Can you work these out from the model? Positions are in its coordinate system, mm. Coordinates: 2 decimals unless noted, no trailing zeros. Loops run counter-clockwise (first coordinate to the right, second up) from the corner with the lowest first, then second, coordinate; pieces in that order, holes last. Notation, with made-up numbers: (-24, -35.75) -> (15, -35.75) arc R33 cw to (15, -0.75) -> close; hole circle Ø11 at (-36.5, 14). An arc over 180 degrees is marked (long way). Use one line per item in the form item = value. Start each with the question number.
(1) Imagine slicing it at A-A (y = -23). List the corners of the cut face in (x, z) for me.
(2) Imagine slicing it at B-B (x = 47.5). List the corners of the cut face in (y, z) for me.
(3) I'm going to push a flat-ended pin straight in: pin 1 (8 mm diameter, centred on x = -12, y = -1.5, fed in from +Z). Where does the tip first touch, or does it pass through?
(4) Imagine slicing it at C-C (z = 1.5). State how many separate pieces and enclosed holes the cut face has, plus the area to 4 significant figures.
(5) Thinking about a two-plate mould opening in Y: for faces 1 (the flat face through (30, 7.5, 3)), 2 (the flat face through (-1, 0, 5)), which applies, released by +Y, released by -Y, zero draft, split by the parting line, or undercut?
(6) I need wall thicknesses on line 1 (Y direction, x = 26, z = 1.75). Which ranges of the line are inside material? Lowest first, please. Write a range as [from, to].
```python
from build123d import *

# Parameters (mm, degrees)
SKETCH_1_W                  = 125
SKETCH_1_H                  = 65
EXTRUDE_1_DEPTH             = 5
SKETCH_2_W                  = 15
SKETCH_2_H                  = 15
CUT_EXTRUDE_1_DEPTH         = 5
PATTERN_LINEAR_1_COUNT      = 6
PATTERN_LINEAR_1_PITCH      = 20
PATTERN_LINEAR_1_COUNT_DIR2 = 3
PATTERN_LINEAR_1_PITCH_DIR2 = 20


with BuildPart() as part:
    # 草图1 → 凸台-拉伸1 (new body)
    with BuildSketch(Plane.XY):
        Rectangle(SKETCH_1_W, SKETCH_1_H)
    extrude(amount=EXTRUDE_1_DEPTH)

    # 草图2 → 切除-拉伸1 (cut)
    with BuildSketch(Plane.XY.offset(5)):
        with Locations((-50, 20)):
            Rectangle(SKETCH_2_W, SKETCH_2_H)
    cut_extrude_1 = extrude(amount=-CUT_EXTRUDE_1_DEPTH, mode=Mode.SUBTRACT)

    # 阵列(线性)1: Cut-Extrude 1 6 × 3
    with Locations(*[(i * PATTERN_LINEAR_1_PITCH, -j * PATTERN_LINEAR_1_PITCH_DIR2, 0) for i in range(PATTERN_LINEAR_1_COUNT) for j in range(PATTERN_LINEAR_1_COUNT_DIR2) if (i, j) != (0, 0)]):
        add(cut_extrude_1, mode=Mode.SUBTRACT)


solid = part.part
```
Worked out:
q1.outline = (-62.5, 0) -> (-57.5, 0) -> (-57.5, 5) -> (-62.5, 5) -> close; (-42.5, 0) -> (-37.5, 0) -> (-37.5, 5) -> (-42.5, 5) -> close; (-22.5, 0) -> (-17.5, 0) -> (-17.5, 5) -> (-22.5, 5) -> close; (-2.5, 0) -> (2.5, 0) -> (2.5, 5) -> (-2.5, 5) -> close; (17.5, 0) -> (22.5, 0) -> (22.5, 5) -> (17.5, 5) -> close; (37.5, 0) -> (42.5, 0) -> (42.5, 5) -> (37.5, 5) -> close; (57.5, 0) -> (62.5, 0) -> (62.5, 5) -> (57.5, 5) -> close
q2.outline = (-32.5, 0) -> (-27.5, 0) -> (-27.5, 5) -> (-32.5, 5) -> close; (-12.5, 0) -> (-7.5, 0) -> (-7.5, 5) -> (-12.5, 5) -> close; (7.5, 0) -> (12.5, 0) -> (12.5, 5) -> (7.5, 5) -> close; (27.5, 0) -> (32.5, 0) -> (32.5, 5) -> (27.5, 5) -> close
q3.pin_1 = through
q4.separate_pieces = 1
q4.enclosed_holes = 18
q4.area = 4,075 mm2
q5.face_1 = undercut
q5.face_2 = zero draft
q6.line_1 = [-32.5, -27.5], [-12.5, -7.5], [7.5, 12.5], [27.5, 32.5]
